Could you check a few things on this model? Use its own coordinates, in mm. A direction names the side the tool comes from. Coordinates: 2 decimals unless noted, no trailing zeros. Order: outer loops, then holes, each group sorted by start corner. A loop starts at its lowest first (then second) coordinate and runs counter-clockwise, first axis right, second up. Notation, with made-up numbers: (35, 23.25) - (46, 23.25) arc R19 ccw to (46, 44.25) - close; hole circle Ø9 at (48, 64.25). An arc over 180 degrees is marked (long way). One line per item, written item: value. Start each with the question number.
Autodesk Inventor part; units mm, degrees
ref_plane "YZ Plane" through (0, 0, 0) normal (1, 0, 0) x (0, 1, 0)
ref_plane "XZ Plane" through (0, 0, 0) normal (0, 1, 0) x (-1, 0, 0)
ref_plane "XY Plane" through (0, 0, 0) normal (0, 0, 1) x (1, 0, 0)
sketch "Sketch1" plane through (0, 0, 0) normal (0, 0, 1) x (1, 0, 0)
  line L0 (-12.6521, 8.2446) -> (12.7479, 8.2446)
  line L1 (12.7479, 8.2446) -> (12.7479, -42.5554)
  line L2 (12.7479, -42.5554) -> (-12.6521, -42.5554)
  line L3 (-12.6521, -42.5554) -> (-12.6521, 8.2446)
  line L4 (9.5729, 5.0696) -> (-9.4771, 5.0696)
  line L5 (-9.4771, 5.0696) -> (-9.4771, -39.3804)
  line L6 (-9.4771, -39.3804) -> (9.5729, -39.3804)
  line L7 (9.5729, -39.3804) -> (9.5729, 5.0696)
  point P0 (0, 0)
  dimension "d1" = 25.4
  dimension "d4" = 50.8
  dimension "d5" = 3.175
extrude "Extrusion1" add sketch "Sketch1" along normal blind 133.35
sketch "Sketch2" plane through (-12.6521, 8.2446, 0) normal (0, 1, 0) x (1, 0, 0)
  line L0 (25.4, 0) -> (25.4, -133.35)
  line L1 (25.4, -133.35) -> (0, -133.35)
  point P0 (12.6521, 0)
  point P1 (12.7, -34.925)
  point P2 (12.7, -98.425)
  dimension "d8" = 63.5
  dimension "d9" = 12.7
  dimension "d10" = 12.7
  dimension "d11" = 34.925
hole "Hole1" at (0.0479, 8.2446, 34.925) at (0.0479, 8.2446, 98.425) direction (0, -1, 0) diameter 6.35 end through all
properties part number "Motor Tension Block Mount"
Q1. I want a section at A-A on x = -7.75. Please give me the cut outline in (y, z), then the cut area to 3 significant figures.
Q2. Which directions (+Z, -Z, +X, -X, +Y, -Y) give clear straight access to the entire face, cutting with the end or side of a thin tool? Please do faces 5 (the cylindrical face through (-0.91, -40.99, 37.95)), 6 (the flat face through (0, -39.38, 66)).
Q3. We'd pull the mould along X, two halves only. Please class faces 1 (the flat face through (12.748, -17, 66)), 2 (the flat face through (0, 5.07, 66)), 3 (the flat face through (-12.652, -18, 66)), 4 (the flat face through (-10, -19, 0)): +X half, -X half, draft (parallel to the pull), parting line (faces both ways), or undercut.
Q4. I want a section at C-C on z = 62.5. Please give me the cut outline in (x, y).
Q5. I want a section at B-B on y = -32.5. Please give me the cut outline in (x, z).
Q6. If I drill on L1, parallel to Y at x = -6.75, z = 50; L2, parallel to X at y = -30.5, z = 51; L3, parallel to X at y = 6.5, z = 32.5, over which ranges is the centre line in solid material (lowest first)?
Values follow:
1. outline: (-42.56, 0) - (-39.38, 0) - (-39.38, 133.35) - (-42.56, 133.35) - close; (5.07, 0) - (8.24, 0) - (8.24, 133.35) - (5.07, 133.35) - close
1. area: 847 mm^2
2. face 5: +Y, -Y
2. face 6: +Z, -Z
3. face 1: +X half
3. face 2: undercut
3. face 3: -X half
3. face 4: draft
4. outline: (-12.65, -42.56) - (12.75, -42.56) - (12.75, 8.24) - (-12.65, 8.24) - close; hole (-9.48, -39.38) - (9.57, -39.38) - (9.57, 5.07) - (-9.48, 5.07) - close
5. outline: (-12.65, 0) - (-9.48, 0) - (-9.48, 133.35) - (-12.65, 133.35) - close; (9.57, 0) - (12.75, 0) - (12.75, 133.35) - (9.57, 133.35) - close
6. L1: y = -42.56 to -39.38, 5.07 to 8.24
6. L2: x = -12.65 to -9.48, 9.57 to 12.75
6. L3: x = -12.65 to -2, 2.1 to 12.75
